Geometry check sheet. Reference: the model listing, model coordinates, mm. A direction names the side the tool comes from. Round coordinates to 2 decimals unless told otherwise and drop trailing zeros. Write each loop counter-clockwise with the first axis right and the second up, starting at its lowest first coordinate (ties: lowest second). Pieces come first, ordered by that corner, then holes. Notation, with made-up numbers: (-1.75, 22) -> (17.25, 22) arc R33 cw to (17.25, 53) -> close; hole circle Ø8 at (66.5, 52). An arc over 180 degrees is marked (long way). Put each result on its own line as item: value. Start each with the question number.
Autodesk Inventor part; units mm, degrees
ref_plane "Work Plane1" through (0, 45, 27) normal (1, 0, 0) x (0, 0, -1)
ref_plane "Work Plane2" through (0, 45, -81) normal (-1, 0, 0) x (0, 0, 1)
ref_plane "YZ Plane" through (0, 0, 0) normal (1, 0, 0) x (0, 1, 0)
sketch "Sketch1" plane through (0, 0, 0) normal (0, 0, 1) x (1, 0, 0)
  line L0 (-31, -31) -> (31, -31)
  line L1 (31, -31) -> (31, 31)
  line L2 (31, 31) -> (-31, 31)
  line L3 (-31, 31) -> (-31, -31)
  line L4 (-31, -31) -> (31, 31) construction
  line L5 (31, -31) -> (-31, 31) construction
  line L6 (-33, 33) -> (33, 33)
  line L7 (33, 33) -> (33, -33)
  line L8 (33, -33) -> (-33, -33)
  line L9 (-33, -33) -> (-33, 33)
  point P0 (0, 0)
  dimension "d0" = 62
  dimension "d1" = 62
  dimension "d2" = 2
extrude "Extrusion1" add sketch "Sketch1" along normal blind 2 contours L3 L2 L1 L0 | L6 L7 L8 L9
extrude "Extrusion2" add sketch "Sketch1" against normal blind 12
sketch "Sketch2" plane through (-33, 33, 2) normal (0, 1, 0) x (1, 0, 0)
  line L0 (13, 3) -> (53, 3)
  line L1 (53, 3) -> (53, 0)
  line L2 (53, 0) -> (13, 0)
  line L3 (13, 0) -> (13, 3)
  line L4 (0, 14) -> (0, 0)
  line L5 (0, 14) -> (66, 14)
  point P0 (33, 2)
  dimension "d7" = 40
  dimension "d8" = 3
  dimension "d9" = 13
  dimension "d10" = 11
extrude "Extrusion3" add sketch "Sketch2" along normal blind 12
sketch "Sketch3" plane through (20, 33, -1) normal (0, 0, -1) x (-1, 0, 0)
  line L0 (40, 12) -> (0, 12)
  line L1 (40, 0) -> (40, 12)
  line L2 (0, 12) -> (40, 12)
  line L3 (40, 12) -> (40, 9)
  line L4 (40, 9) -> (0, 9)
  line L5 (0, 9) -> (0, 12)
  point P0 (20, -33)
  dimension "d13" = 3
extrude "Extrusion4" add sketch "Sketch3" along normal blind 80
sketch "Sketch4" plane through (-20, 42, -1) normal (0, -1, 0) x (1, 0, 0)
  line L0 (30.5, -63) -> (9.5, -63)
  line L1 (9.5, -63) -> (9.5, -22)
  line L2 (9.5, -22) -> (30.5, -22)
  line L3 (30.5, -22) -> (30.5, -63)
  line L4 (40, 3) -> (40, -80)
  line L5 (0, 3) -> (40, 3)
  point P0 (20, 1)
  dimension "d16" = 21
  dimension "d17" = 41
  dimension "d18" = 9.5
  dimension "d19" = 25
extrude "Extrusion5" cut sketch "Sketch4" against normal blind 80
sketch "Sketch5" plane through (-20, 42, -1) normal (0, -1, 0) x (1, 0, 0)
  line L0 (30.5, -63) -> (9.5, -63)
  line L1 (30.5, -63) -> (9.5, -63)
  line L2 (9.5, -63) -> (9.5, -70)
  line L3 (9.5, -70) -> (30.5, -70)
  line L4 (30.5, -70) -> (30.5, -63)
  circle A0 centre (15, -66.75) radius 2.25
  line L5 (30.5, -22) -> (30.5, -63)
  line L6 (30.5, -22) -> (9.5, -22)
  line L7 (9.5, -22) -> (9.5, -15)
  line L8 (9.5, -15) -> (30.5, -15)
  line L9 (30.5, -15) -> (30.5, -22)
  circle A1 centre (25, -18.5) radius 2.25
  point P0 (20, 1)
  point P1 (14.9217, -69.81)
  point P2 (13.9783, -69.81)
  point P3 (25.0283, -15.19)
  point P4 (25.9717, -15.19)
  dimension "d22" = 7
  dimension "d23" = 4.5
  dimension "d24" = 3.75
  dimension "d25" = 5.5
  dimension "d26" = 7
  dimension "d27" = 4.5
  dimension "d28" = 5.5
  dimension "d29" = 3.5
extrude "Extrusion6" cut sketch "Sketch5" against normal blind 80 contours A0 | A1
sketch "Sketch6" plane through (-33, -33, 2) normal (0, -1, 0) x (1, 0, 0)
  line L0 (0, -14) -> (0, 0)
  line L1 (66, -14) -> (66, 0)
  line L2 (0, 0) -> (66, 0)
  line L3 (66, 0) -> (66, -14)
  line L4 (66, -14) -> (0, -14)
  line L5 (0, -14) -> (0, 0)
  point P0 (33, -2)
  point P1 (66, 0)
extrude "Extrusion7" cut sketch "Sketch6" against normal up to surface (75 mm away)
sketch "Sketch7" plane through (0, 0, 2) normal (0, 0, 1) x (1, 0, 0)
  line L0 (-20, 42) -> (-20, 45)
  line L1 (20, 42) -> (20, 45)
  line L2 (-20, 45) -> (20, 45)
  line L3 (20, 45) -> (20, 42)
  line L4 (20, 42) -> (-20, 42)
  line L5 (-20, 42) -> (-20, 45)
  point P0 (0, 0)
extrude "Extrusion8" add sketch "Sketch7" along normal blind 25
sketch "Sketch8" plane through (-20, 42, -81) normal (0, -1, 0) x (1, 0, 0)
  line L0 (0, 108) -> (0, 0)
  line L1 (40, 0) -> (40, 108)
  line L2 (0, 108) -> (40, 108)
  line L3 (40, 108) -> (40, 105)
  line L4 (40, 105) -> (0, 105)
  line L5 (0, 105) -> (0, 108)
  point P0 (20, 81)
  dimension "d36" = 3
extrude "Extrusion9" add sketch "Sketch8" along normal blind 100
sketch "Sketch9" plane through (20, 42, 24) normal (0, 0, -1) x (-1, 0, 0)
  circle A0 centre (20, -90) radius 2
  circle A1 centre (8, -50) radius 2
  circle A2 centre (32, -20) radius 2
  line L0 (40, 0) -> (40, -100)
  line L1 (0, 0) -> (0, -100)
  line L2 (40, -100) -> (0, -100)
  line L3 (0, 0) -> (40, 0)
  point P0 (20, -42)
  dimension "d39" = 4
  dimension "d40" = 4
  dimension "d41" = 4
  dimension "d42" = 8
  dimension "d43" = 8
  dimension "d44" = 20
  dimension "d45" = 10
  dimension "d46" = 50
  dimension "d47" = 20
extrude "Extrusion10" cut sketch "Sketch9" against normal blind 10 contours A0 | A1 | A2
ref_plane "Work Plane1" through (0, 45, 27) normal (1, 0, 0) x (0, 0, -1)
sketch "Sketch11" plane through (20, 45, 27) normal (1, 0, 0) x (0, 0, -1)
  line L0 (3, -3) -> (3, -103)
  line L1 (3, -3) -> (103, -3)
  line L2 (103, -3) -> (103, -19)
  line L3 (103, -19) -> (3, -19)
  line L4 (3, -19) -> (3, -3)
  line L5 (103, -3) -> (3, -19)
  point P0 (27, -45)
  point P1 (3, -19)
  dimension "d55" = 100
  dimension "d56" = 16
extrude "Extrusion12" add sketch "Sketch11" against normal blind 4 contours L1 L5 L0
ref_plane "Work Plane2" through (0, 45, -81) normal (-1, 0, 0) x (0, 0, 1)
mirror "Mirror1" about plane through (0, 45, -81) normal (-1, 0, 0) of "Extrusion12"
sketch "Sketch12" plane through (-20, -58, -81) normal (0, -1, 0) x (1, 0, 0)
  line L0 (0, 108) -> (0, 0)
  line L1 (40, 0) -> (40, 108)
  line L2 (0, 108) -> (40, 108)
  line L3 (40, 108) -> (40, 105)
  line L4 (40, 105) -> (0, 105)
  line L5 (0, 105) -> (0, 108)
  point P0 (20, 81)
  dimension "d59" = 3
extrude "Extrusion13" cut sketch "Sketch12" against normal blind 40
sketch "Sketch13" plane through (20, 26, 24) normal (0, 0, -1) x (-1, 0, 0)
  circle A0 centre (32, -34) radius 2
  line L0 (0, -44) -> (40, -44)
  line L1 (40, 0) -> (40, -44)
  point P0 (20, -26)
  dimension "d62" = 4
  dimension "d63" = 10
  dimension "d64" = 8
extrude "Extrusion14" cut sketch "Sketch13" against normal blind 40
sketch "Sketch14" plane through (0, 0, 27) normal (0, 0, 1) x (1, 0, 0)
  line L0 (-20, 45) -> (20, 45)
  line L1 (-20, 45) -> (-8, 45)
  line L2 (-8, 45) -> (-8, 29)
  line L3 (-8, 29) -> (-20, 29)
  line L4 (-20, 29) -> (-20, 45)
  point P0 (0, 0)
  dimension "d67" = 12
  dimension "d68" = 16
extrude "Extrusion15" cut sketch "Sketch14" against normal blind 10
properties part number "pan_base_holder_first_v1"
(1) Sectioned sample at B-B (x = 12). Record the cut outline in (y, z), and give its area (3 significant figures).
(2) Material ranges on L1, parallel to Z at x = 5, y = 44.25; L2, parallel to Y at x = -12, z = 24.85; L3, parallel to Z at x = -5, y = 43.25, recorded low to high. Write a range as from..to.
(3) Sectioned sample at D-D (x = 5). Record the cut outline in (y, z).
(4) Sectioned sample at C-C (y = 22). Record the cut outline in (x, z).
(5) Sectioned sample at A-A (z = -50). Record the cut outline in (x, y).
(6) Set-up check for faces 5 (the flat face through (16, 36, -14)), 6 (the flat face through (0, -18, 26)), 7 (the flat face through (10.5, 43, -43)), 8 (the flat face through (-17, 39, 17)), 9 (the cylindrical face through (-10, -8, 25)): record each of +Z, -Z, +X, -X, +Y, -Y from which the full face is reachable in a straight line by a thin tool's end or side.
(7) Mould release check, pull along X, two halves, no side actions. Record for faces 1 (the flat face through (20, 35, -7)), 2 (the flat face through (0, 42, -18)), 3 (the flat face through (-8, 38.9, 24.3)), 4 (the flat face through (-18.03, 33.89, -25.3)): +X half, -X half, draft (parallel to the pull), parting line (faces both ways), or undercut.
(8) Go/stop test with flat-tipped pins: pin 1 Ø3 at (x, z) = (-17, 23) entering from +Y; pin 2 Ø1 at (x, z) = (-16, -25) entering from -Y; pin 3 Ø3 at (x, y) = (-12, -8) entering from +Z; pin 4 Ø1 at (x, y) = (16, 7) entering from -Z. Record where each tip stops, or that it passes through.
Found:
1. outline: (-18, 24) -> (-10, 24) -> (-10, 27) -> (-18, 27) -> close; (-6, 24) -> (42, 24) -> (42, -81) -> (45, -81) -> (45, 27) -> (-6, 27) -> close
1. area: 492 mm2
2. L1: -81..-64, -23..-21.75, -17.25..27
2. L2: -18..-10, -6..20, 24..29
2. L3: -81..-70, -65.5..-64, -23..27
3. outline: (-18, 24) -> (42, 24) -> (42, -17.25) -> (45, -17.25) -> (45, 27) -> (-18, 27) -> close; (42, -81) -> (45, -81) -> (45, -64) -> (42, -64) -> close; (42, -23) -> (45, -23) -> (45, -21.75) -> (42, -21.75) -> close
4. outline: (-20, 24) -> (-14, 24) -> (-14, 27) -> (-20, 27) -> close; (-10, 24) -> (20, 24) -> (20, 27) -> (-10, 27) -> close
5. outline: (-20, 37.84) -> (-16, 37.84) -> (-16, 42) -> (-10.5, 42) -> (-10.5, 45) -> (-20, 45) -> close; (10.5, 42) -> (16, 42) -> (16, 37.84) -> (20, 37.84) -> (20, 45) -> (10.5, 45) -> close
6. face 5: -Z, -Y
6. face 6: +Z, -Z, +X, -X, -Y
6. face 7: +Y, -Y
6. face 8: +Z, -X, +Y
6. face 9: +Z, -Z
7. face 1: +X half
7. face 2: undercut
7. face 3: -X half
7. face 4: draft
8. pin 1: y = 29
8. pin 2: y = 33.76
8. pin 3: through
8. pin 4: z = 24
